CAD build for the part. Positions are in the model's coordinates, mm. A direction names the side the tool comes from. Round coordinates to 2 decimals unless told otherwise and drop trailing zeros. Write each loop counter-clockwise with the first axis right and the second up, starting at its lowest first coordinate (ties: lowest second). Pieces come first, ordered by that corner, then holes. Notation, with made-up numbers: (30.25, 76.5) - (63.25, 76.5) arc R17 cw to (63.25, 87.5) - close; hole circle Ø3 at (63, -31.75). An arc over 180 degrees is marked (long way). Put each result on its own line as item: value. Start each with the question number.
Item 1: Mould opens along Z. For faces 5 (the flat face through (40, 19, 10)), 6 (the cylindrical face through (80.43, 1.39, 10.45)), 7 (the flat face through (47, 9, 20)), 8 (the flat face through (23, 9.5, 10)) say: released by +Z, released by -Z, zero draft, split by the parting line, or undercut.
Item 2: Pin check, flat tips, straight feed: pin 1 Ø2.5 at (x, z) = (79, 10) entering from +Y (1 decimal); pin 2 Ø3 at (x, z) = (24, 6) entering from +Y; pin 3 Ø5 at (x, z) = (24.5, 6.5) entering from -Y; pin 4 Ø12 at (x, z) = (49.5, 11) entering from +Y. Stop position of each tip, or through.
Item 3: Cut at D-D (x = 71). Give the cut face in (y, z).
Item 4: Cut at C-C (z = 5.75). Give the cut face in (x, y), and give its area (3 significant figures).
Item 5: Cut at B-B (x = 79). Give the cut face in (y, z).
Item 6: 3-axis set-ups, long thin cutter, end or side, ignore diameter. For faces 1 (the flat face through (21, 5, 10)), 2 (the flat face through (41, 0, 10)), 3 (the flat face through (81, 11.5, 10)), 4 (the flat face through (30, 19, 10)): which of +Z, -Z, +X, -X, +Y, -Y reach the whole face in a straight line?
Item 7: Drill centre lines: line 1 (Z direction, x = 25, y = 14); line 2 (X direction, y = 16.5, z = 4); line 3 (X direction, y = 13.5, z = 10.75). Where is each one in solid material? Low to high. Write a range as from..to.
Item 8: Cut at A-A (y = 15). Give the cut face in (x, z), and give its area (3 significant figures).
Autodesk Fusion 360 part; units mm, degrees
sketch "Sketch1" plane through (0, 0, 0) normal (0, 0, 1) x (1, 0, 0)
  line L0 (25, 0) -> (25, 21)
  line L1 (25, 21) -> (46, 21)
  line L2 (46, 21) -> (46, 0)
  line L3 (46, 0) -> (25, 0)
  line L4 (35.5, 21) -> (35.5, 19)
  line L5 (35.5, 0) -> (35.5, 2)
  line L6 (25, 10.5) -> (28, 10.5)
  line L7 (25, 19) -> (35.5, 19)
  line L8 (25, 2) -> (35.5, 2)
  line L9 (28, 21) -> (28, 0)
  line L10 (35.5, 19) -> (35.5, 2)
  line L11 (28, 10.5) -> (35.5, 10.5)
  circle A0 centre (35.5, 10.5) radius 8.5
  line L12 (44, 10.5) -> (47.291, 10.5)
  line L13 (47.291, 10.5) -> (61.791, 10.5)
  circle A1 centre (61.791, 10.5) radius 14.5
  circle A2 centre (61.791, 10.5) radius 17
  line L14 (46, 21) -> (48.4213, 21)
  line L15 (46, 0) -> (48.4213, 0)
  line L16 (61.791, 10.5) -> (61.791, 27.5)
  line L17 (61.791, 10.5) -> (61.791, -6.5)
  line L18 (61.791, -6.5) -> (79.291, -6.5)
  line L19 (61.791, 27.5) -> (79.291, 27.5)
  line L20 (79.291, 27.5) -> (79.291, -6.5)
  line L21 (79.291, 27.5) -> (76.291, 27.5)
  line L22 (76.291, 27.5) -> (76.291, 11.5)
  line L23 (76.291, 11.5) -> (79.291, 11.5)
  line L24 (76.291, -6.5) -> (76.291, 9.5)
  line L25 (76.291, 9.5) -> (79.291, 9.5)
  line L26 (27, 10.5) -> (24, 10.5)
  line L27 (25, 21) -> (24, 21)
  line L28 (24, 21) -> (24, 11.5)
  line L29 (24, 11.5) -> (25, 11.5)
  line L30 (24, 0) -> (24, 9.5)
  line L31 (24, 9.5) -> (25, 9.5)
  line L32 (25, 0) -> (24, 0)
  dimension "d1" = 21
  dimension "d2" = 21
  dimension "d4" = 3
  dimension "d5" = 17
  dimension "d6" = 3.291
  dimension "d7" = 14.5
  dimension "d8" = 34
  dimension "d9" = 17.5
  dimension "d10" = 17.5
  dimension "d11" = 3
  dimension "d12" = 16
  dimension "d13" = 16
  dimension "d14" = 9.5
  dimension "d15" = 9.5
extrude "Extrude1" add sketch "Sketch1" along normal blind 20
extrude "Extrude2" cut sketch "Sketch1" along normal blind 24 contours L9 L10 L11 A0 | L10 A0 | L6 L9 A0 | L6 L9 A0 | L9 L10 L11 A0 | L13 A1 L16 | L13 A1 L17 | A1 L16 L17
box "BoxPrimitive1" cut length 2 width 3.1 height 22 placed x (0, -1, 0) y (1, 0, 0) z (0, 0, 1) at (76.2, 11.5, 0)
box "BoxPrimitive2" cut length 2 width 3.5 height 21 placed x (0, -1, 0) y (1, 0, 0) z (0, 0, 1) at (24, 11.5, 0)
sketch "Sketch8" plane through (0, 21, 0) normal (0, 1, 0) x (-1, 0, 0)
  line L0 (-48.4213, 0) -> (-24, 0)
  line L1 (-24, 0) -> (-24, 20)
  line L2 (-24, 20) -> (-48.4213, 20)
  line L3 (-48.4213, 20) -> (-48.4213, 0)
  line L4 (-30, 5) -> (-30, 15)
  line L5 (-40, 5) -> (-40, 15)
  spline S0 degree 5 poles (-30, 5) (-30.2, 4.7725) (-30.6, 4.3372) (-31.2, 3.744) (-32, 3.0743) (-33, 2.4528) (-34, 2.0663) (-35, 1.934) (-36, 2.0663) (-37, 2.4528) (-38, 3.0743) (-38.8, 3.744) (-39.4, 4.3372) (-39.8, 4.7725) (-40, 5) knots 0 0 0 0 0 0 0.1 0.2 0.3 0.4 0.5 0.6 0.7 0.8 0.9 1 1 1 1 1 1
  spline S1 degree 5 poles (-30, 15) (-30.2, 15.2275) (-30.6, 15.6628) (-31.2, 16.256) (-32, 16.9257) (-33, 17.5472) (-34, 17.9337) (-35, 18.066) (-36, 17.9337) (-37, 17.5472) (-38, 16.9257) (-38.8, 16.256) (-39.4, 15.6628) (-39.8, 15.2275) (-40, 15) knots 0 0 0 0 0 0 0.1 0.2 0.3 0.4 0.5 0.6 0.7 0.8 0.9 1 1 1 1 1 1
  point P0 (-35, 2)
  point P1 (-35, 18)
extrude "Extrude3" add 2 faces at (24, 14.6667, 13.3333) (24, 3.1667, 6.6667) along direction (-1, 0, 0) blind 3
cylinder "CylinderPrimitive3" cut diameter 3 height -23 placed x (1, 0, 0) y (0, 0, -1) z (0, 1, 0) at (25, 21, 10)
extrude "Extrude4" cut sketch "Sketch8" against normal blind 24 contours L4 L5 S0 S1
extrude "Extrude5" add 2 faces at (79.291, 4.1667, 6.6667) (79.291, 22.1667, 6.6667) along direction (1, 0, 0) blind 3
cylinder "CylinderPrimitive4" cut diameter 3 height -36 placed x (1, 0, 0) y (0, 0, 1) z (0, -1, 0) at (79, -6.5, 10)
Output values:
1. face 5: undercut
1. face 6: undercut
1. face 7: released by +Z
1. face 8: zero draft
2. pin 1: through
2. pin 2: y = 21
2. pin 3: y = 0
2. pin 4: y = 26.29
3. outline: (-6.5, 0) - (-0.7, 0) - (-0.7, 20) - (-6.5, 20) - close; (21.7, 0) - (27.5, 0) - (27.5, 20) - (21.7, 20) - close
4. outline: (21, 0) - (30, 0) - (30, 4.02) arc R8.5 cw to (27.06, 9.5) - (21, 9.5) - close; (21, 11.5) - (27.06, 11.5) arc R8.5 cw to (30, 16.98) - (30, 21) - (21, 21) - close; (40, 0) - (48.42, 0) arc R17 ccw to (61.79, -6.5) - (82.29, -6.5) - (82.29, 9.5) - (76.26, 9.5) arc R14.5 cw (long way) to (76.26, 11.5) - (82.29, 11.5) - (82.29, 27.5) - (61.79, 27.5) arc R17 ccw to (48.42, 21) - (40, 21) - (40, 17.71) arc R8.5 cw to (40, 3.29) - close
4. area: 712 mm2
5. outline: (-6.5, 0) - (9.5, 0) - (9.5, 8.5) - (-6.5, 8.5) - close; (-6.5, 11.5) - (9.5, 11.5) - (9.5, 20) - (-6.5, 20) - close; (11.5, 0) - (27.5, 0) - (27.5, 8.5) - (11.5, 8.5) - close; (11.5, 11.5) - (27.5, 11.5) - (27.5, 20) - (11.5, 20) - close
6. face 1: +Z, -Z, -X, +Y, -Y
6. face 2: +Z, -Z, -X, -Y
6. face 3: +Z, -Z, +X
6. face 4: +Y, -Y
7. line 1: 0..8.5, 11.5..20
7. line 2: 21..29.48, 41.52..48.59, 74.99..82.29
7. line 3: 21..23.7, 26.3..27.55, 43.45..47.6, 75.98..77.7, 80.3..82.29
8. outline: (21, 0) - (28.29, 0) - (28.29, 20) - (21, 20) - close; (42.71, 0) - (48.01, 0) - (48.01, 20) - (42.71, 20) - close; (75.58, 0) - (82.29, 0) - (82.29, 20) - (75.58, 20) - close; hole circle Ø3 at (25, 10); hole circle Ø3 at (79, 10)
8. area: 372 mm2
